```python
from build123d import *

# Parameters (mm, degrees)
F0_W      = 30
F0_H      = 30
F1_DEPTH  = 900
F2_W      = 30
F2_H      = 30
F3_DEPTH  = 2300
F4_W      = 30
F4_H      = 10
F5_DEPTH  = 65
F6_W      = 40
F6_H      = 16
F7_DEPTH  = 760.001
F9_W      = 1.5
F9_H      = 800
F10_DEPTH = 2330


with BuildPart() as f1:
    # F0 (on Top) → F1 (new body)
    with BuildSketch(Plane.XY):
        with Locations((-1150, 0)):
            Rectangle(F0_W, F0_H)
        with Locations((1150, 0)):
            Rectangle(F0_W, F0_H)
    extrude(amount=-F1_DEPTH)

    # F2 (on face) → F3 (join, through all)
    with BuildSketch(Plane.YZ.offset(1165)):
        with Locations((0, -15)):
            Rectangle(F2_W, F2_H)
        with Locations((0, -405)):
            Rectangle(F2_W, F2_H)
        with Locations((0, -785)):
            Rectangle(F2_W, F2_H)
    extrude(amount=-F3_DEPTH)

    # F8: F5 across plane


with BuildPart() as f5:
    # F4 (on face) → F5 (new body)
    with BuildSketch(Plane.YZ.offset(1165)):
        with Locations((0, -145)):
            Rectangle(F4_W, F4_H)
        with Locations((0, -745)):
            Rectangle(F4_W, F4_H)
    extrude(amount=F5_DEPTH)

    # F6 (on face) → F7 (cut, through all)
    with BuildSketch(Plane.XY.offset(-140)):
        with BuildLine():
            Line((1230, 15), (1227.360249, 15))
            ThreePointArc((1227.360249, 15), (1229.33503, 7.615252), (1230, 0))
            Line((1230, 0), (1230, 15))
        make_face()
        with BuildLine():
            ThreePointArc((1230, 0), (1229.33503, -7.615253), (1227.360249, -15))
            Line((1227.360249, -15), (1230, -15))
            Line((1230, -15), (1230, 0))
        make_face()
        with Locations((1200, 0)):
            Rectangle(F6_W, F6_H)
        with BuildLine():
            Line((1220, 8), (1220, -8))
            ThreePointArc((1220, -8), (1223.450166, 0), (1220, 8))
        make_face()
        with BuildLine():
            ThreePointArc((1180, 8), (1176.549834, 0), (1180, -8))
            Line((1180, -8), (1180, 8))
        make_face()
    extrude(amount=-F7_DEPTH, mode=Mode.SUBTRACT)


with BuildPart() as f1_1:
    add(f1.part)
    add(f5.part.mirror(Plane.YZ))


    add(f5.part)  # F10 merges F5
    # F9 (on face) → F10 (join, through all)
    with BuildSketch(Plane.YZ.offset(1165)):
        with Locations((15.75, -400)):
            Rectangle(F9_W, F9_H)
    extrude(amount=-F10_DEPTH)


solid = f1_1.part
```
Check sheet for the modelled part. Datum: model origin and axes. Units: mm. A direction names the side the tool comes from. Round coordinates to 2 decimals unless told otherwise and drop trailing zeros. Loops run counter-clockwise (first coordinate to the right, second up) from the corner with the lowest first, then second, coordinate; pieces in that order, holes last. Notation, with made-up numbers: (58, 42.5) - (70, 42.5) arc R17 ccw to (70, 72.5) - close; hole circle Ø3 at (-10.5, 84.25). An arc over 180 degrees is marked (long way). Write item = value, one per line. Start each with the question number.
Q1. Access from +Z, -Z, +X, -X, +Y, -Y to the whole of each face (thin tool, end or side, straight path). Record for faces 1 (the face through (16, 15, -597)), 2 (the face through (-6, -15, -415)).
Q2. Release check for a two-part mould opening along X. For faces 3 (the face through (16, 16.5, -406)), 4 (the face through (16, 15, -213)) record: pulls with the +X half, pulls with the -X half, needs draft (parallel to the pull), parting line crosses it, or undercut.
Q3. Section check A-A (x = -102.5). Record the boundary of the cut face in (y, z), plus the area to 3 significant figures.
Q4. Thickness scan on L1, parallel to Z at x = 490, y = -8.5; L2, parallel to X at y = -5.5, z = -604.5; L3, parallel to X at y = 14, z = -798. Record the ranges inside material, lowest first.
Q5. Section check B-B (z = -215). Record the boundary of the cut face in (x, y).
Q6. Depth check by flat-ended pin: P1, Ø3, axis at x = 1196.5, z = -146, coming from the +Y side; P2, Ø15, axis at x = 1212, y = 3.5, coming from the +Z side; P3, Ø5, axis at y = 7, z = -790.5, coming from the -X side; P4, Ø9, axis at x = -1196.5, y = -0.5, coming from the -Z side. Enter the tip coordinate at first touch or a pass-through.
Derived:
q1.face_1 = -Y
q1.face_2 = +Z, -Z, +X, -X, -Y
q2.face_3 = needs draft
q2.face_4 = undercut
q3.outline = (-15, -800) - (16.5, -800) - (16.5, 0) - (-15, 0) - (-15, -30) - (15, -30) - (15, -390) - (-15, -390) - (-15, -420) - (15, -420) - (15, -770) - (-15, -770) - close
q3.area = 3,900 mm^2
q4.L1 = -800 to -770, -420 to -390, -30 to 0
q4.L2 = -1165 to -1135, 1135 to 1165
q4.L3 = -1165 to 1165
q5.outline = (-1165, -15) - (-1135, -15) - (-1135, 15) - (1135, 15) - (1135, -15) - (1165, -15) - (1165, 16.5) - (-1165, 16.5) - close
q6.P1 = 15
q6.P2 = -140
q6.P3 = -1165
q6.P4 = through
